Verification items for the finished model (mm, model axes). A direction names the side the tool comes from. Round coordinates to 2 decimals unless told otherwise and drop trailing zeros. Loops run counter-clockwise (first coordinate to the right, second up) from the corner with the lowest first, then second, coordinate; pieces in that order, holes last. Notation, with made-up numbers: (30.25, -5) -> (75.25, -5) arc R21 ccw to (75.25, 32) -> close; hole circle Ø1 at (56, 52.5). An arc over 180 degrees is marked (long way). Write item = value, one per line.
```python
from build123d import *

# Parameters (mm, degrees)
SKETCH_1_R      = 20
SKETCH_1_R_2    = 13
SKETCH_1_R_3    = 1.7
SKETCH_1_R_4    = 1.75
EXTRUDE_1_DEPTH = 15


with BuildPart() as part:
    # 草图1 → 凸台-拉伸1 (new body)
    with BuildSketch(Plane(origin=(0, 0, 0), x_dir=(1, 0, 0), z_dir=(0, 1, 0))):
        with BuildLine():
            Line((65.196415688, 20.938478113), (339.27978891, 27.990735896))
            ThreePointArc((339.27978891, 27.990735896), (368, 0), (339.27978891, -27.990735896))
            Line((339.27978891, -27.990735896), (65.196415688, -20.938478113))
            ThreePointArc((65.196415688, -20.938478113), (39.495702891, -23.306065445), (15.054107063, -31.597054618))
            ThreePointArc((15.054107063, -31.597054618), (-35, 0), (15.054107063, 31.597054618))
            ThreePointArc((15.054107063, 31.597054618), (39.495702891, 23.306065445), (65.196415688, 20.938478113))
        make_face()
        with Locations(Location((0, 0, 0), (0, 0, 270))):
            Circle(SKETCH_1_R, mode=Mode.SUBTRACT)
        with Locations(Location((340, 0, 0), (0, 0, 270))):
            Circle(SKETCH_1_R_2, mode=Mode.SUBTRACT)
        with Locations(Location((340, 21, 0), (0, 0, 270))):
            Circle(SKETCH_1_R_3, mode=Mode.SUBTRACT)
        with Locations(Location((358.186533479, 10.5, 0), (0, 0, 270))):
            Circle(SKETCH_1_R_3, mode=Mode.SUBTRACT)
        with Locations(Location((358.186533479, -10.5, 0), (0, 0, 270))):
            Circle(SKETCH_1_R_3, mode=Mode.SUBTRACT)
        with Locations(Location((340, -21, 0), (0, 0, 270))):
            Circle(SKETCH_1_R_3, mode=Mode.SUBTRACT)
        with Locations(Location((321.813466521, -10.5, 0), (0, 0, 270))):
            Circle(SKETCH_1_R_3, mode=Mode.SUBTRACT)
        with Locations(Location((321.813466521, 10.5, 0), (0, 0, 270))):
            Circle(SKETCH_1_R_3, mode=Mode.SUBTRACT)
        with Locations(Location((0, 28.5, 0), (0, 0, 270))):
            Circle(SKETCH_1_R_4, mode=Mode.SUBTRACT)
        with Locations(Location((-24.681724008, 14.25, 0), (0, 0, 270))):
            Circle(SKETCH_1_R_4, mode=Mode.SUBTRACT)
        with Locations(Location((-24.681724008, -14.25, 0), (0, 0, 270))):
            Circle(SKETCH_1_R_4, mode=Mode.SUBTRACT)
        with Locations(Location((0, -28.5, 0), (0, 0, 270))):
            Circle(SKETCH_1_R_4, mode=Mode.SUBTRACT)
        with Locations(Location((24.681724008, -14.25, 0), (0, 0, 270))):
            Circle(SKETCH_1_R_4, mode=Mode.SUBTRACT)
        with Locations(Location((24.681724008, 14.25, 0), (0, 0, 270))):
            Circle(SKETCH_1_R_4, mode=Mode.SUBTRACT)
    extrude(amount=EXTRUDE_1_DEPTH)


solid = part.part
```
(1) Sectioned sample at C-C, the plane x = 218. Record the cut outline in (y, z), and give its area (3 significant figures).
Filled sheet:
outline = (0, -24.87) -> (15, -24.87) -> (15, 24.87) -> (0, 24.87) -> close
area = 746 mm2
(2) Material ranges on probe 1 along X at (y, z) = (5.5, -10.5); probe 2 along X at (y, z) = (8.25, 0); probe 3 along X at (y, z) = (3, -7) (3 decimals), recorded low to high. Write a range as from..to.
Filled sheet:
probe_1 = -33.39..-17.02, 17.02..320.11, 323.51..332.34, 347.66..356.49, 359.89..365.96
probe_2 = -35..-20, 20..327, 353..368
probe_3 = -34.293..-18.735, 18.735..329.046, 350.954..367.111
(3) Go/stop test with flat-tipped pins: pin 1 Ø8 at (y, z) = (9.5, -1) entering from -X; pin 2 Ø1 at (x, y) = (197.5, 4) entering from +Z; pin 3 Ø1 at (x, z) = (223.5, 21.5) entering from -Y; pin 4 Ø2 at (x, z) = (24.68, -14.25) entering from -Y. Record where each tip stops, or that it passes through.
Filled sheet:
pin_1 = -35
pin_2 = 24.36
pin_3 = 0
pin_4 = through
(4) Sectioned sample at D-D, the plane x = 109.5. Record the cut outline in (y, z).
Filled sheet:
outline = (0, -22.08) -> (15, -22.08) -> (15, 22.08) -> (0, 22.08) -> close
(5) Sectioned sample at A-A, the plane z = 0. Record the cut outline in (x, y), and give its area (4 significant figures).
Filled sheet:
outline = (-35, 0) -> (-20, 0) -> (-20, 15) -> (-35, 15) -> close; (20, 0) -> (327, 0) -> (327, 15) -> (20, 15) -> close; (353, 0) -> (368, 0) -> (368, 15) -> (353, 15) -> close
area = 5,055 mm2
(6) Sectioned sample at B-B, the plane y = 2.75. Count the separate pieces of the cut face and the enclosed holes in it, and give its area (3 significant figures).
Filled sheet:
separate_pieces = 1
enclosed_holes = 14
area = 18,200 mm2
(7) Set-up check for faces 4 (the face through (39.85, 7.4, 23.23)), 5 (the face through (-19.524, 7.395, -4.336)): record each of +Z, -Z, +X, -X, +Y, -Y from which the full face is reachable in a straight line by a thin tool's end or side.
Filled sheet:
face_4 = +Z, +Y, -Y
face_5 = +Y, -Y
(8) Draft check along X on faces 1 (the face through (-34.986, 7.395, 0.987)), 2 (the face through (39.142, 7.395, -23.382)), 3 (the face through (169, 0, 0)). Enter one of: released by +X, released by -X, zero draft, split by the parting line, or undercut.
Filled sheet:
face_1 = split by the parting line
face_2 = undercut
face_3 = zero draft
